Verification items for the finished model (mm, model axes). A direction names the side the tool comes from. Give positions to 0.01 mm unless a question says otherwise; leave off trailing zeros. Order: outer loops, then holes, each group sorted by start corner. A loop starts at its lowest first (then second) coordinate and runs counter-clockwise, first axis right, second up. Notation, with made-up numbers: (79.25, 58) -> (98.25, 58) arc R23 ccw to (98.25, 83) -> close; hole circle Ø11 at (62.5, 14.5). An arc over 180 degrees is marked (long way). Return JSON: item names as keys, results as strings. Group by question number.
(1) Cross-section at B-B on x = 136. Enter the section's corners in (y, z) (3 decimals), then the cut area to 3 significant figures.
(2) Cross-section at A-A on z = 199. Enter the section's corners in (x, y) (3 decimals).
(3) Tool access check on faces 4 (the face through (158.4, 0, 202)), 5 (the face through (151.875, -1.597, 161.953)), 6 (the face through (153, 0, 222.25)), 7 (the face through (166, 0, 215.25)). Record the directions out of +Z, -Z, +X, -X, +Y, -Y that give a thin tool (end or side, any length) a straight path to the whole face; none if there is none.
(4) Release check for a two-part mould opening along X. For faces 1 (the face through (149.08, -0.04, 170.71)), 2 (the face through (179.865, -0.044, 196.494)), 3 (the face through (152.95, -0.044, 146.456)) record: pulls with the +X half, pulls with the -X half, needs draft (parallel to the pull), parting line crosses it, or undercut.
(5) Depth check by flat-ended pin: pin 1 Ø2 at (x, z) = (141.38, 165.54) entering from -Y; pin 2 Ø0.8 at (x, y) = (125.5, -0.5) entering from +Z; pin 3 Ø2.5 at (x, y) = (166.4, 0) entering from +Z; pin 4 Ø4.5 at (x, z) = (163.02, 164.86) entering from -Y (3 decimals). Enter the tip coordinate at first touch or a pass-through.
(6) Thickness scan on line 1 along Z through (x, y) = (164, -0.5); line 2 along X through (y, z) = (-0.5, 170); line 3 along Z through (x, y) = (155, 2.5). Record the ranges inside material, lowest first.
from build123d import *

# Parameters (mm, degrees)
PLACA_ANTEBRAZO_START          = -3.175
PLACA_ANTEBRAZO_DEPTH          = 6.35
PLACA_ANTEBRAZO_REDONDEO_START = -3.175
CROQUIS13_R                    = 25
PLACA_ANTEBRAZO_REDONDEO_DEPTH = 6.35
BARRENOS_J3_START              = -3.175
CROQUIS14_R                    = 1.7
CROQUIS14_R_2                  = 2.05
CROQUIS14_R_3                  = 3.4
BARRENOS_J3_DEPTH              = 6.35
REFRENTADOS_J3_START           = -3.175
CROQUIS15_R                    = 3
REFRENTADOS_J3_DEPTH           = 3.2
ALIGERADO_PASO_CABLE_START     = -3.175
ALIGERADO_PASO_CABLE_DEPTH     = 6.35
ROSCA_M3_CANTO_START           = 213.25
CROQUIS17_R                    = 1.25
ROSCA_M3_CANTO_DEPTH           = 9
PASADORES_D3_START             = 215.25
CROQUIS18_R                    = 1.5
PASADORES_D3_DEPTH             = 7
PASO_M3_BASES_CINCHO_START     = -3.175
CROQUIS20_R                    = 1.7
PASO_M3_BASES_CINCHO_DEPTH     = 6.35


with BuildPart() as part:
    # Croquis12 → Placa_antebrazo (new body)
    with BuildSketch(Plane(origin=(0, 0, 0), x_dir=(1, 0, 0), z_dir=(0, 1, 0)).offset(PLACA_ANTEBRAZO_START)):
        Polygon((127.4, -171.45), (177.4, -171.45), (182.4, -222.25), (122.4, -222.25), align=None)
    extrude(amount=PLACA_ANTEBRAZO_DEPTH)

    # Croquis13 → Placa_antebrazo_redondeo (add)
    with BuildSketch(Plane(origin=(0, 0, 0), x_dir=(1, 0, 0), z_dir=(0, 1, 0)).offset(PLACA_ANTEBRAZO_REDONDEO_START)):
        with Locations((152.4, -171.45)):
            Circle(CROQUIS13_R)
    extrude(amount=PLACA_ANTEBRAZO_REDONDEO_DEPTH)

    # Croquis14 → Barrenos_J3 (cut)
    with BuildSketch(Plane(origin=(0, 0, 0), x_dir=(1, 0, 0), z_dir=(0, 1, 0)).offset(BARRENOS_J3_START)):
        with Locations(Location((163.416293151, -177.356884561, 0), (0, 0, 270))):
            Circle(CROQUIS14_R)
        with Locations(Location((152.792634488, -183.943832005, 0), (0, 0, 270))):
            Circle(CROQUIS14_R)
        with Locations(Location((141.776341338, -178.036947444, 0), (0, 0, 270))):
            Circle(CROQUIS14_R)
        with Locations(Location((141.383706849, -165.543115439, 0), (0, 0, 270))):
            Circle(CROQUIS14_R)
        with Locations(Location((152.007365512, -158.956167995, 0), (0, 0, 270))):
            Circle(CROQUIS14_R)
        with Locations(Location((163.023658662, -164.863052556, 0), (0, 0, 270))):
            Circle(CROQUIS14_R)
        with Locations(Location((157.774949114, -180.118905468, 0), (0, 0, 270))):
            Circle(CROQUIS14_R_2)
        with Locations(Location((142.205033084, -171.770389743, 0), (0, 0, 270))):
            Circle(CROQUIS14_R_2)
        with Locations(Location((157.220017802, -162.460704789, 0), (0, 0, 270))):
            Circle(CROQUIS14_R_2)
        with Locations(Location((152.4, -171.45, 0), (0, 0, 270))):
            Circle(CROQUIS14_R_3)
    extrude(amount=BARRENOS_J3_DEPTH, mode=Mode.SUBTRACT)

    # Croquis15 → Refrentados_J3 (cut)
    with BuildSketch(Plane(origin=(0, 0, 0), x_dir=(1, 0, 0), z_dir=(0, 1, 0)).offset(REFRENTADOS_J3_START)):
        with Locations(Location((163.416293151, -177.356884561, 0), (0, 0, 90))):
            Circle(CROQUIS15_R)
        with Locations(Location((152.792634488, -183.943832005, 0), (0, 0, 90))):
            Circle(CROQUIS15_R)
        with Locations(Location((141.776341338, -178.036947444, 0), (0, 0, 90))):
            Circle(CROQUIS15_R)
        with Locations(Location((141.383706849, -165.543115439, 0), (0, 0, 90))):
            Circle(CROQUIS15_R)
        with Locations(Location((152.007365512, -158.956167995, 0), (0, 0, 90))):
            Circle(CROQUIS15_R)
        with Locations(Location((163.023658662, -164.863052556, 0), (0, 0, 90))):
            Circle(CROQUIS15_R)
    extrude(amount=REFRENTADOS_J3_DEPTH, mode=Mode.SUBTRACT)

    # Croquis16 → Aligerado_paso_cable (cut)
    with BuildSketch(Plane(origin=(0, 0, 0), x_dir=(1, 0, 0), z_dir=(0, 1, 0)).offset(ALIGERADO_PASO_CABLE_START)):
        with BuildLine():
            Line((158.4, -195), (158.4, -210))
            ThreePointArc((158.4, -210), (152.4, -216), (146.4, -210))
            Line((146.4, -210), (146.4, -195))
            ThreePointArc((146.4, -195), (152.4, -189), (158.4, -195))
        make_face()
    extrude(amount=ALIGERADO_PASO_CABLE_DEPTH, mode=Mode.SUBTRACT)

    # Croquis17 → Rosca_M3_canto (cut)
    with BuildSketch(Plane.XY.offset(ROSCA_M3_CANTO_START)):
        with Locations((125.4, 0)):
            Circle(CROQUIS17_R)
        with Locations((179.4, 0)):
            Circle(CROQUIS17_R)
    extrude(amount=ROSCA_M3_CANTO_DEPTH, mode=Mode.SUBTRACT)

    # Croquis18 → Pasadores_D3 (cut)
    with BuildSketch(Plane.XY.offset(PASADORES_D3_START)):
        with Locations((138.4, 0)):
            Circle(CROQUIS18_R)
        with Locations((166.4, 0)):
            Circle(CROQUIS18_R)
    extrude(amount=PASADORES_D3_DEPTH, mode=Mode.SUBTRACT)

    # Croquis20 → Paso_M3_bases_cincho (cut)
    with BuildSketch(Plane(origin=(0, 0, 0), x_dir=(1, 0, 0), z_dir=(0, 1, 0)).offset(PASO_M3_BASES_CINCHO_START)):
        with Locations(Location((168.9, -211, 0), (0, 0, 270))):
            Circle(CROQUIS20_R)
    extrude(amount=PASO_M3_BASES_CINCHO_DEPTH, mode=Mode.SUBTRACT)


solid = part.part
Verdict:
{
 "1": {"outline": "(-3.175, 152.581) -> (3.175, 152.581) -> (3.175, 222.25) -> (-3.175, 222.25) -> close", "area": "442 mm²"},
 "2": {"outline": "(124.688, -3.175) -> (146.4, -3.175) -> (146.4, 3.175) -> (124.688, 3.175) -> close; (158.4, -3.175) -> (180.112, -3.175) -> (180.112, 3.175) -> (158.4, 3.175) -> close"},
 "3": {"face 4": "+Y, -Y", "face 5": "-Y", "face 6": "+Z, +X, -X, +Y, -Y", "face 7": "+Z"},
 "4": {"face 1": "undercut", "face 2": "pulls with the +X half", "face 3": "parting line crosses it"},
 "5": {"pin 1": "through", "pin 2": "z = 213.25", "pin 3": "z = 215.25", "pin 4": "y = 0.025"},
 "6": {"line 1": "149.3 to 162.03, 167.7 to 174.41, 180.3 to 222.25", "line 2": "127.44 to 141.17, 143.24 to 149.32, 155.48 to 177.36", "line 3": "146.59 to 169.26, 173.64 to 189.59, 215.41 to 222.25"}
}
